For this review, take the finished solid that the model builds, in its own axes (mm). A direction names the side the tool comes from. Coordinates: 2 decimals unless noted, no trailing zeros. Loops run counter-clockwise (first coordinate to the right, second up) from the corner with the lowest first, then second, coordinate; pieces in that order, holes last. Notation, with made-up numbers: (11, 74) -> (33, 74) arc R31 ccw to (33, 99) -> close; hole circle Ø1 at (50, 71.5). An arc over 180 degrees is marked (long way). Answer in a Markdown table with one row per item.
from build123d import *

# Parameters (mm, degrees)
F0_R      = 30
F1_DEPTH  = 15
F2_R      = 26.5
F3_DEPTH  = 8
F4_R      = 20
F5_DEPTH  = 40
F6_R      = 20
F7_DEPTH  = 7
F9_DEPTH  = 1
F11_DEPTH = 25
F12_R     = 5
F13_SIZE2 = 10
F13_SIZE  = 5
F14_R     = 1
F15_DEPTH = 15
F16_R     = 4.7918026285
F16_R_2   = 1
F17_DEPTH = 22
F18_R     = 27.5
F18_R_2   = 4.7918026285
F19_DEPTH = 25


# Not quite as in the source:
# - a feature names something its author has since deleted; it is built from what else it names


with BuildPart() as f1:
    # F0 (on Top) → F1 (new body)
    with BuildSketch(Plane.XY):
        Circle(F0_R)
    extrude(amount=F1_DEPTH)

    # F2 (on face) → F3 (join)
    with BuildSketch(Plane.XY.offset(15)):
        Circle(F2_R)
    extrude(amount=F3_DEPTH)

    # F4 (on face) → F5 (join)
    with BuildSketch(Plane.XY.offset(23)):
        Circle(F4_R)
    extrude(amount=F5_DEPTH)

    # F6 (on face) → F7 (join)
    with BuildSketch(Plane(origin=(0, 0, 0), x_dir=(1, 0, 0), z_dir=(0, 0, -1))):
        Circle(F6_R)
    extrude(amount=F7_DEPTH)

    # F8 (on Right) → F9 (join)
    with BuildSketch(Plane.YZ):
        with BuildLine():
            Line((37.5, 0.200964841), (0, 0.200964841))
            Line((0, 0.200964841), (0, -19.799035159))
            Line((0, -19.799035159), (35, -19.799035159))
            ThreePointArc((35, -19.799035159), (40.3033008589, -17.6023360179), (42.5, -12.299035159))
            Line((42.5, -12.299035159), (42.5, -4.799035159))
            ThreePointArc((42.5, -4.799035159), (41.0355339059, -1.2635012531), (37.5, 0.200964841))
        make_face()
        with BuildLine():
            Line((0, -19.799035159), (0, 0.200964841))
            Line((0, 0.200964841), (-37.5, 0.200964841))
            ThreePointArc((-37.5, 0.200964841), (-41.0355339059, -1.2635012531), (-42.5, -4.799035159))
            Line((-42.5, -4.799035159), (-42.5, -12.299035159))
            ThreePointArc((-42.5, -12.299035159), (-40.3033008589, -17.6023360179), (-35, -19.799035159))
            Line((-35, -19.799035159), (0, -19.799035159))
        make_face()
    extrude(amount=F9_DEPTH)

    # F10 (on face) → F11 (cut)
    with BuildSketch(Plane.YZ.offset(1)):
        with BuildLine():
            Line((-23.7842038121, -19.799035159), (23.7842038121, -19.799035159))
            ThreePointArc((23.7842038121, -19.799035159), (0, -12.2829212631), (-23.7842038121, -19.799035159))
        make_face()
    extrude(amount=-F11_DEPTH, mode=Mode.SUBTRACT)

    # F12
    f12_edges = [f1.edges().sort_by_distance(p)[0] for p in [
        (0.5, -23.784204, -19.799035),
        (0.5, 23.784204, -19.799035),
    ]]
    fillet(f12_edges, radius=F12_R)

    # F13
    f13_edges = [f1.edges().sort_by_distance(p)[0] for p in [
        (-20, 0, 63),
    ]]
    f13_side = f1.faces().sort_by_distance((0, 0, 63))[0]
    chamfer(f13_edges, length=F13_SIZE, length2=F13_SIZE2, reference=f13_side)

    # F14 (on face) → F15 (join)
    with BuildSketch(Plane.XY.offset(63)):
        Circle(F14_R)
    extrude(amount=F15_DEPTH)

    # F16 (on face) → F17 (join)
    with BuildSketch(Plane.XY.offset(63)):
        Circle(F16_R)
        Circle(F16_R_2, mode=Mode.SUBTRACT)
        Circle(F16_R_2)
    extrude(amount=F17_DEPTH)

    # F18 (on face) → F19 (join)
    with BuildSketch(Plane.XY.offset(85)):
        Circle(F18_R)
        Circle(F18_R_2, mode=Mode.SUBTRACT)
        Circle(F18_R_2)
    extrude(amount=F19_DEPTH)


solid = f1.part
Item 1: For L1, parallel to Z at x = 3.5, y = 5; L2, parallel to Z at x = -14, y = 22; L3, parallel to Z at x = 4, y = 2, list the stretches that pass through material, from the lowest coordinate up.
Worked answers:
| item | result |
|---|---|
| L1 | -7 to 63, 85 to 110 |
| L2 | 0 to 23, 85 to 110 |
| L3 | -7 to 110 |
Item 2: Take a section at B-B, the plane z = 10.5. State the section outline as (x, y) points.
Worked answers:
| item | result |
|---|---|
| outline | circle Ø60 at (0, 0) |
Item 3: Take a section at C-C, the plane z = 34.5. State the section outline as (x, y) points, and give its area (3 significant figures).
Worked answers:
| item | result |
|---|---|
| outline | circle Ø40 at (0, 0) |
| area | 1,260 mm² |
Item 4: Insertion check: pin 1 (10 mm diameter, centred on x = -0.5, z = 88, fed in from +Y); pin 2 (9 mm diameter, centred on x = -22, y = 4.5, fed in from -Z); pin 3 (1.5 mm diameter, centred on y = -22.5, z = 96.5, fed in from +X). Each pin has a flat end and moves straight along its axis. Give the tip position at first contact, or say it passes through.
Worked answers:
| item | result |
|---|---|
| pin 1 | y = 27.5 |
| pin 2 | z = -7 |
| pin 3 | x = 16.83 |
Item 5: For faces 1 (the cylindrical face through (-3.8, -2.92, 73.85)), 2 (the cylindrical face through (0.493, -40.361, -17.544)), 3 (the flat face through (-22, 0, 0)), 4 (the flat face through (8, 0, -7)), 5 (the flat face through (22, 0, 0)), list the 3-axis set-ups (+Z, -Z, +X, -X, +Y, -Y) from which the entire face can be reached by the end or side of a thin tool; tool diameter is ignored.
Worked answers:
| item | result |
|---|---|
| face 1 | none |
| face 2 | -Z, +X, -X, -Y |
| face 3 | -Z, -X |
| face 4 | -Z, +X, +Y, -Y |
| face 5 | -Z, +X |
Item 6: The part is to be moulded in two halves that separate along Z. For faces 6 (the cylindrical face through (-4.336, -19.524, 37.79)), 7 (the cylindrical face through (0.49, 41.07, -1.3)), 8 (the cylindrical face through (20, 0, -3)), say which applies: +Z half, -Z half, draft (parallel to the pull), parting line (faces both ways), or undercut.
Worked answers:
| item | result |
|---|---|
| face 6 | undercut |
| face 7 | +Z half |
| face 8 | draft |
